```python
from build123d import *

# Parameters (mm, degrees)
ESQUISSE1_R             = 6.4135
BOSS_EXTRU_1_DEPTH      = 6.35
ESQUISSE5_R             = 8.255
ENL_V_MAT_EXTRU_3_DEPTH = 7.35


with BuildPart() as part:
    # Esquisse1 → Boss.-Extru.1 (new body)
    with BuildSketch(Plane.XY):
        with BuildLine():
            Line((-3.81, -14.6685), (-3.81, -60.96))
            ThreePointArc((-3.81, -60.96), (-1.950128061, -65.450128061), (2.54, -67.31))
            Line((2.54, -67.31), (15.811710267, -67.31))
            ThreePointArc((15.811710267, -67.31), (18.15660317, -67.758815604), (20.170023782, -69.041818182))
            ThreePointArc((20.170023782, -69.041818182), (33.02, -63.5), (20.170023782, -57.958181818))
            ThreePointArc((20.170023782, -57.958181818), (18.15660317, -59.241184396), (15.811710267, -59.69))
            Line((15.811710267, -59.69), (10.16, -59.69))
            ThreePointArc((10.16, -59.69), (5.669871939, -57.830128061), (3.81, -53.34))
            Line((3.81, -53.34), (3.81, -14.6685))
            ThreePointArc((3.81, -14.6685), (4.534969751, -11.722055584), (6.544341637, -9.448393238))
            ThreePointArc((6.544341637, -9.448393238), (0, 11.4935), (-6.544341637, -9.448393238))
            ThreePointArc((-6.544341637, -9.448393238), (-4.534969751, -11.722055584), (-3.81, -14.6685))
        make_face()
        Circle(ESQUISSE1_R, mode=Mode.SUBTRACT)
        with Locations((25.4, -63.5)):
            Circle(ESQUISSE1_R, mode=Mode.SUBTRACT)
    extrude(amount=BOSS_EXTRU_1_DEPTH)

    # Esquisse5 → Enlèv. mat.-Extru.3 (cut, through all)
    with BuildSketch(Plane(origin=(0, 0, 0), x_dir=(-1, 0, 0), z_dir=(0, 0, -1))):
        with Locations((-1.254065113, -71.897575416)):
            Circle(ESQUISSE5_R)
    extrude(amount=-ENL_V_MAT_EXTRU_3_DEPTH, mode=Mode.SUBTRACT)


solid = part.part
```
Geometry: final body of the model. Coordinates: model frame, mm. A direction names the side the tool comes from. Coordinates: 2 decimals unless noted, no trailing zeros. Write each loop counter-clockwise with the first axis right and the second up, starting at its lowest first coordinate (ties: lowest second). Pieces come first, ordered by that corner, then holes. Notation, with made-up numbers: M 73.5,71.5 L 77.5,71.5 A21 cw 77.5,75.5 Z; hole C -28,-6 d1. An arc over 180 degrees is marked long. Use CSV: the item, a comma, the result in double quotes. Start each with the question number.
1. First-contact query: P1, Ø2, axis at y = -3.5, z = 1.5, coming from the +X side; P2, Ø2, axis at y = -52, z = 3, coming from the +X side; P3, Ø2, axis at x = 11.5, z = 3.5, coming from the -Y side. Flat tips, straight axial feed; report the tip coordinate or a pass-through.
2. Cut plane C-C on z = 5.5. Count the separate pieces of the cut face and the enclosed holes in it, plus the area to 3 significant figures.
3. Ray query, probe 1 along X at (y, z) = (-59, 5); probe 2 along Y at (x, z) = (25.4, 3); probe 3 along Y at (x, z) = (22, 3.75). Return the intervals inside material, ascending.
4. Mould query, pull axis Y, two halves, no side actions, for faces 5 (the face through (12, -67.31, 3)), 6 (the face through (18.188, -59.229, 3.131)), 7 (the face through (5.72, -57.88, 3.13)), 8 (the face through (2, -33, 0)). Classes: pulls with the +Y half, pulls with the -Y half, needs draft (parallel to the pull), parting line crosses it, or undercut.
5. Cut plane A-A on y = 0. Return the cut outline in (x, z).
6. Cut plane D-D on y = -15.5. Return the cut outline in (x, z), plus the area to 3 significant figures.
7. Cut plane B-B on x = 25.4. Return the cut outline in (y, z).
8. Reachability of faces 1 (the face through (3.17, -63.87, 3.13)), 2 (the face through (13, -59.69, 3)), 3 (the face through (-3.81, -37, 3)), 4 (the face through (3.81, -34, 3)) from +Z, -Z, +X, -X, +Y, -Y: full face, straight path, thin tool, end or side. Return the list, or none.
Entries:
1,P1,"x = 11.22"
1,P2,"x = 3.81"
1,P3,"y = -67.31"
2,separate pieces,"1"
2,enclosed holes,"2"
2,area,"855 mm²"
3,probe 1,"-3.81 to 7.28, 18.69 to 20.83, 29.97 to 31.55"
3,probe 2,"-71.12 to -69.91, -57.09 to -55.88"
3,probe 3,"-70.32 to -68.94, -58.06 to -56.68"
4,face 5,"pulls with the -Y half"
4,face 6,"pulls with the +Y half"
4,face 7,"undercut"
4,face 8,"needs draft"
5,outline,"M -11.49,0 L -6.41,0 L -6.41,6.35 L -11.49,6.35 Z; M 6.41,0 L 11.49,0 L 11.49,6.35 L 6.41,6.35 Z"
6,outline,"M -3.81,0 L 3.81,0 L 3.81,6.35 L -3.81,6.35 Z"
6,area,"48.4 mm²"
7,outline,"M -71.12,0 L -69.91,0 L -69.91,6.35 L -71.12,6.35 Z; M -57.09,0 L -55.88,0 L -55.88,6.35 L -57.09,6.35 Z"
8,face 1,"+Z, -Z, -Y"
8,face 2,"+Z, -Z"
8,face 3,"+Z, -Z, -X, -Y"
8,face 4,"+Z, -Z, +X"
